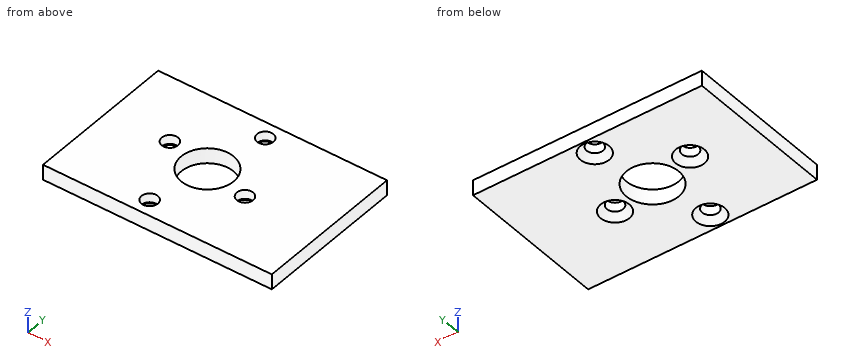
from build123d import *

# Parameters (mm, degrees)
SKETCH1_W           = 47.6504
SKETCH1_H           = 31.3182
SKETCH1_R           = 1.7
SKETCH1_R_2         = 5.461
BOSS_EXTRUDE1_DEPTH = 3.175
CHAMFER1_SIZE       = 1.29999994


with BuildPart() as part:
    # Sketch1 → Boss-Extrude1 (new body)
    with BuildSketch(Plane.XY):
        with Locations((1.5748, 0)):
            Rectangle(SKETCH1_W, SKETCH1_H)
        with Locations((9.336418849, -1.984517089)):
            Circle(SKETCH1_R, mode=Mode.SUBTRACT)
        with Locations((-9.336418849, 1.984517089)):
            Circle(SKETCH1_R, mode=Mode.SUBTRACT)
        with Locations((2.613449954, 12.295315341)):
            Circle(SKETCH1_R, mode=Mode.SUBTRACT)
        with Locations((-2.613449954, -12.295315341)):
            Circle(SKETCH1_R, mode=Mode.SUBTRACT)
        Circle(SKETCH1_R_2, mode=Mode.SUBTRACT)
    extrude(amount=BOSS_EXTRUDE1_DEPTH)

    # Chamfer1
    chamfer1_edges = [part.edges().sort_by_distance(p)[0] for p in [
        (7.636418849, -1.984517089, 0),
        (-11.036418849, 1.984517089, 0),
        (0.913449954, 12.295315341, 0),
        (-4.313449954, -12.295315341, 0),
    ]]
    chamfer(chamfer1_edges, length=CHAMFER1_SIZE)


solid = part.part
Source: CAD feature listing. Evaluate the final solid. Frame: model axes, mm. Round coordinates to 2 decimals unless told otherwise and drop trailing zeros. Loops run counter-clockwise (first coordinate to the right, second up) from the corner with the lowest first, then second, coordinate; pieces in that order, holes last.
Q1. First-contact query: P1, Ø4.5, axis at x = -9.34, y = 1.98, coming from the -Z side. Flat tip, straight axial feed; report the tip coordinate or a pass-through.
Q2. Ray query, line 1 (X direction, y = -2.5, z = 2.5); line 2 (X direction, y = 3, z = 0.2); line 3 (Y direction, x = 2.5, z = 0.45). Return the intervals inside material, ascending.
Q3. Section A-A, the plane z = 2.45. Return loops of the section in (x, y), plus the area to 3 significant figures.
Solutions:
1. P1: stops at z = 0.74
2. line 1: x = -22.25 to -4.86, 4.86 to 7.72, 10.96 to 25.4
2. line 2: x = -22.25 to -11.95, -6.73 to -4.56, 4.56 to 25.4
2. line 3: y = -15.66 to -4.86, 4.86 to 9.75, 14.84 to 15.66
3. outline: (-22.25, -15.66) - (25.4, -15.66) - (25.4, 15.66) - (-22.25, 15.66) - close; hole circle Ø3.4 at (-9.34, 1.98); hole circle Ø10.92 at (0, 0); hole circle Ø3.4 at (-2.61, -12.3); hole circle Ø3.4 at (2.61, 12.3); hole circle Ø3.4 at (9.34, -1.98)
3. area: 1,360 mm2
